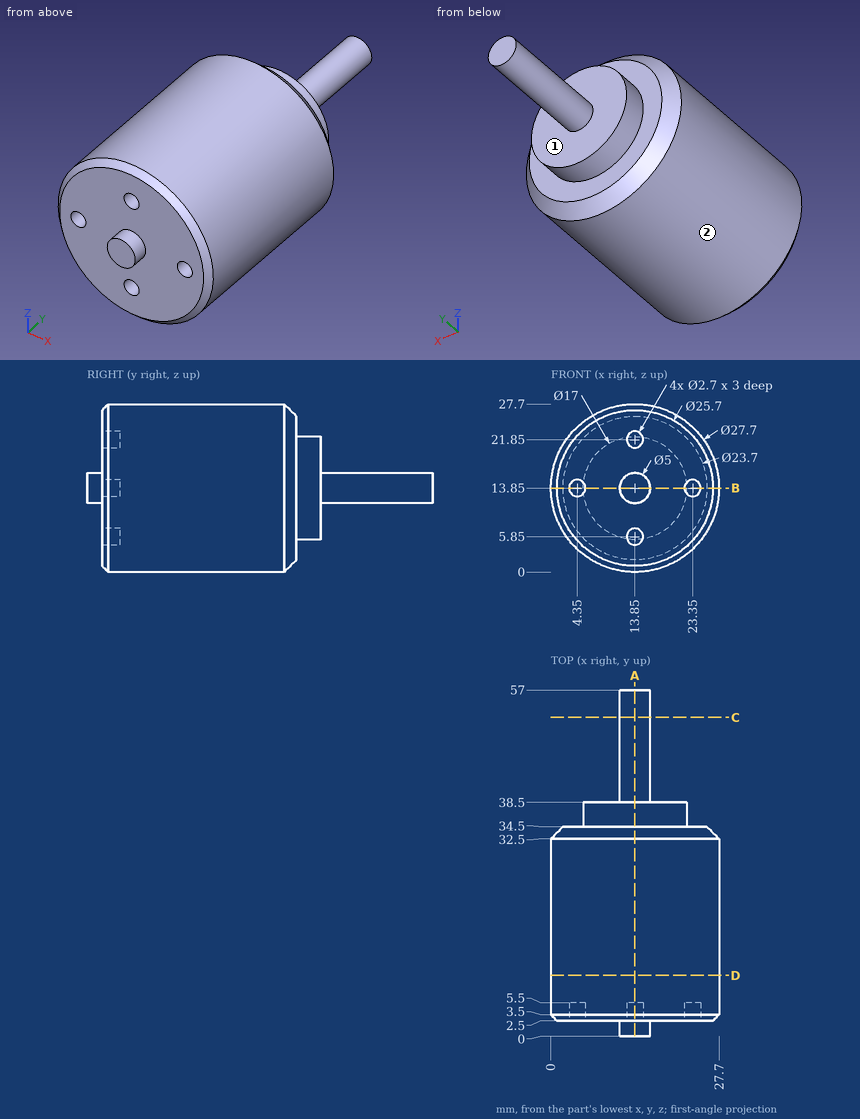
Drawing for the job (mm, zero at the part's lowest x, y, z). A direction names the side the tool comes from. Round coordinates to 2 decimals unless told otherwise and drop trailing zeros. Loops run counter-clockwise (first coordinate to the right, second up) from the corner with the lowest first, then second, coordinate; pieces in that order, holes last. Notation, with made-up numbers: (-3, 70.25) -> (11, 70.25) arc R31 ccw to (11, 98.25) -> close; hole circle Ø2 at (65, -11). An arc over 180 degrees is marked (long way). Answer as CSV lines item,"result". Start each with the question number.
1) Pin check, flat tips, straight feed: P1, Ø2, axis at x = 14, z = 22.5, coming from the -Y side; P2, Ø1.6, axis at x = 4.35, z = 13.85, coming from the +Y side; P3, Ø2.5, axis at x = 23.35, z = 13.85, coming from the +Y side; P4, Ø5, axis at x = 12.5, z = 11, coming from the +Y side. Stop position of each tip, or through.
2) Slice it at D-D (y = 10). List the corners of the cut face in (x, z).
3) Slice it at A-A (x = 13.85). List the corners of the cut face in (y, z).
4) Probe line 1 along X through (y, z) = (3.8, 13.85); line 2 along Z through (x, y) = (13, 4); line 3 along Y through (x, z) = (19.5, 18.75). List the from-to ranges inside material, lowest first.
5) Slice it at C-C (y = 52.5). List the corners of the cut face in (x, z).
6) Slice it at B-B (z = 13.85). List the corners of the cut face in (x, y).
7) Tool access for the marked faces 1 and 2: list every direction of +Z, -Z, +X, -X, +Y, -Y with a clear straight run to the whole face (end or side of a thin tool).
Filled in:
1,P1,"stops at y = 2.5"
1,P2,"stops at y = 34.5"
1,P3,"stops at y = 38.5"
1,P4,"stops at y = 57"
2,outline,"circle Ø27.7 at (13.85, 13.85)"
3,outline,"(0, 11.35) -> (2.5, 11.35) -> (2.5, 7.2) -> (5.5, 7.2) -> (5.5, 4.5) -> (2.5, 4.5) -> (2.5, 1) -> (3.5, 0) -> (32.5, 0) -> (34.5, 2) -> (34.5, 5.35) -> (38.5, 5.35) -> (38.5, 11.35) -> (57, 11.35) -> (57, 16.35) -> (38.5, 16.35) -> (38.5, 22.35) -> (34.5, 22.35) -> (34.5, 25.7) -> (32.5, 27.7) -> (3.5, 27.7) -> (2.5, 26.7) -> (2.5, 23.2) -> (5.5, 23.2) -> (5.5, 20.5) -> (2.5, 20.5) -> (2.5, 16.35) -> (0, 16.35) -> close"
4,line 1,"x = 0 to 3, 5.7 to 22, 24.7 to 27.7"
4,line 2,"z = 0.03 to 4.8, 6.9 to 20.8, 22.9 to 27.67"
4,line 3,"y = 2.5 to 38.5"
5,outline,"circle Ø5 at (13.85, 13.85)"
6,outline,"(0, 3.5) -> (1, 2.5) -> (3, 2.5) -> (3, 5.5) -> (5.7, 5.5) -> (5.7, 2.5) -> (11.35, 2.5) -> (11.35, 0) -> (16.35, 0) -> (16.35, 2.5) -> (22, 2.5) -> (22, 5.5) -> (24.7, 5.5) -> (24.7, 2.5) -> (26.7, 2.5) -> (27.7, 3.5) -> (27.7, 32.5) -> (25.7, 34.5) -> (22.35, 34.5) -> (22.35, 38.5) -> (16.35, 38.5) -> (16.35, 57) -> (11.35, 57) -> (11.35, 38.5) -> (5.35, 38.5) -> (5.35, 34.5) -> (2, 34.5) -> (0, 32.5) -> close"
7,face 1,"+Y"
7,face 2,"+Y, -Y"
